Geometry check sheet. Reference: the model listing, model coordinates, mm. A direction names the side the tool comes from. Coordinates: 2 decimals unless noted, no trailing zeros. Order: outer loops, then holes, each group sorted by start corner. A loop starts at its lowest first (then second) coordinate and runs counter-clockwise, first axis right, second up. Notation, with made-up numbers: M 12,-35 L 23,-35 A18 cw 23,-1 Z; hole C 81,31.25 d3. An arc over 180 degrees is marked long. Use CSV: the item, a comma, the result in double quotes. Start each with the question number.
```python
from build123d import *

# Parameters (mm, degrees)
BOSS_EXTRUDE1_DEPTH = 6.35
BOSS_EXTRUDE2_DEPTH = 7.62
BOSS_EXTRUDE3_DEPTH = 19.05
FILLET1_R           = 10.16


with BuildPart() as part:
    # Sketch1 → Boss-Extrude1 (new body)
    with BuildSketch(Plane.XY):
        Polygon((0, 0), (76.2, 0), (76.2, -50.8), (29.329393675, -50.8), align=None)
    extrude(amount=BOSS_EXTRUDE1_DEPTH)

    # Sketch2 → Boss-Extrude2 (add)
    with BuildSketch(Plane.XY):
        Polygon((76.2, 0), (0, 0), (2.932939367, -5.08), (76.2, -5.08), align=None)
    extrude(amount=-BOSS_EXTRUDE2_DEPTH)

    # Sketch3 → Boss-Extrude3 (add)
    with BuildSketch(Plane.XY.offset(6.35)):
        Polygon((29.329393675, -50.8), (35.679393675, -50.8), (6.35, 0), (0, 0), align=None)
    extrude(amount=BOSS_EXTRUDE3_DEPTH)

    # Fillet1
    fillet1_edges = [part.edges().sort_by_distance(p)[0] for p in [
        (21.014696837, -25.4, 6.35),
    ]]
    fillet(fillet1_edges, radius=FILLET1_R)


solid = part.part
```
1) Gauge pin test, flat ends, axial feed: P1, Ø1, axis at y = -24, z = 14, coming from the +X side; P2, Ø4, axis at x = 67, y = -32.5, coming from the -Z side; P3, Ø1, axis at x = 37, z = 18, coming from the -Y side; P4, Ø6, axis at x = 55, z = -5.5, coming from the -Y side. Record the tip position at first contact, or that the pin passes through.
2) Set-up check for faces 3 (the face through (54, -25, 6.35)), 4 (the face through (48, -28, 0)), 5 (the face through (18, -25, 25.4)): record each of +Z, -Z, +X, -X, +Y, -Y from which the full face is reachable in a straight line by a thin tool's end or side.
3) Section check B-B on z = 17.5. Record the boundary of the cut face in (x, y), then the cut area to 3 significant figures.
4) Material ranges on line 1 along Z through (x, y) = (25, -9); line 2 along Z through (x, y) = (45, -4.5); line 3 along X through (y, z) = (-42, 1.5), recorded low to high.
5) Section check C-C on z = -4. Record the boundary of the cut face in (x, y), then the cut area to 3 significant figures.
6) Draft check along X on faces 1 (the face through (21.22, -25.756, 20.893)), 2 (the face through (39, 0, 1)). Enter one of: +X half, -X half, draft (parallel to the pull), parting line (faces both ways), or undercut.
7) Section check A-A on x = 51.5. Record the boundary of the cut face in (y, z), then the cut area to 3 significant figures.
Results are:
1,P1,"stops at x = 20.9"
1,P2,"stops at z = 0"
1,P3,"passes through"
1,P4,"stops at y = -5.08"
2,face 3,"+Z, +X, +Y"
2,face 4,"-Z, +X, -X, -Y"
2,face 5,"+Z, +X, -X, +Y, -Y"
3,outline,"M 0,0 L 29.33,-50.8 L 35.68,-50.8 L 6.35,0 Z"
3,area,"323 mm²"
4,line 1,"z = 0 to 6.35"
4,line 2,"z = -7.62 to 6.35"
4,line 3,"x = 24.25 to 76.2"
5,outline,"M 0,0 L 2.93,-5.08 L 76.2,-5.08 L 76.2,0 Z"
5,area,"380 mm²"
6,face 1,"+X half"
6,face 2,"draft"
7,outline,"M -50.8,0 L -5.08,0 L -5.08,-7.62 L 0,-7.62 L 0,6.35 L -50.8,6.35 Z"
7,area,"361 mm²"
